Source: CAD feature listing. Evaluate the final solid. Frame: model axes, mm. A direction names the side the tool comes from. Round coordinates to 2 decimals unless told otherwise and drop trailing zeros. Write each loop counter-clockwise with the first axis right and the second up, starting at its lowest first coordinate (ties: lowest second). Pieces come first, ordered by that corner, then holes.
from build123d import *

# Parameters (mm, degrees)
F0_W     = 152.4
F0_H     = 127
F1_DEPTH = 50.8
F3_DEPTH = 101.6
F5_DEPTH = 25.4
F6_W     = 127
F6_H     = 50.8
F7_DEPTH = 127


with BuildPart() as f1:
    # F0 (on Front) → F1 (new body)
    with BuildSketch(Plane.XZ):
        with Locations((-6.594061, 23.633106)):
            Rectangle(F0_W, F0_H)
    extrude(amount=F1_DEPTH)

    # F2 (on face) → F3 (join)
    with BuildSketch(Plane.XZ.offset(50.8)):
        Polygon((18.805939, -14.466894), (69.605939, -14.466894), (69.605939, 87.133106), (-57.394061, 87.133106), (-57.394061, 61.733106), (18.805939, 61.733106), align=None)
    extrude(amount=F3_DEPTH)

    # F4 (on face) → F5 (join)
    with BuildSketch(Plane.XY.offset(87.133106)):
        Polygon((69.605939, 0), (-82.794061, 0), (-82.794061, -50.8), (-57.394061, -50.8), (-57.394061, -152.4), (69.605939, -152.4), align=None)
    extrude(amount=F5_DEPTH)

    # F6 (on face) → F7 (join)
    with BuildSketch(Plane.XY.offset(112.533106)):
        with Locations((6.105939, -127)):
            Rectangle(F6_W, F6_H)
    extrude(amount=F7_DEPTH)


solid = f1.part
1) Section query C-C on y = -57.5. Return the cut outline in (x, z), then the cut area to 3 significant figures.
Taken from the geometry:
outline: (-57.39, 61.73) - (18.81, 61.73) - (18.81, -14.47) - (69.61, -14.47) - (69.61, 112.53) - (-57.39, 112.53) - close
area: 10,300 mm2
2) Section query D-D on x = -61. Return the cut outline in (y, z).
Taken from the geometry:
outline: (-50.8, -39.87) - (0, -39.87) - (0, 112.53) - (-50.8, 112.53) - close
3) Material intervals for line 1 (Z direction, x = -25, y = -20.5); line 2 (Y direction, x = -71, z = -28); line 3 (X direction, y = -113.5, z = 3), sorted ascending.
Taken from the geometry:
line 1: z = -39.87 to 112.53
line 2: y = -50.8 to 0
line 3: x = 18.81 to 69.61
4) Reachability of faces 1 (the face through (-57.394, -114, 130)), 2 (the face through (5, -101.6, 175)), 3 (the face through (18.806, -101, 24)) from +Z, -Z, +X, -X, +Y, -Y: full face, straight path, thin tool, end or side. Return the list, or none.
Taken from the geometry:
face 1: +Z, -Z, -X, -Y
face 2: +Z, +X, -X, +Y
face 3: -Z, -X, -Y
5) Section query B-B on z = -9. Return the cut outline in (x, y).
Taken from the geometry:
outline: (-82.79, -50.8) - (18.81, -50.8) - (18.81, -152.4) - (69.61, -152.4) - (69.61, 0) - (-82.79, 0) - close
6) Section query A-A on x = -4. Return the cut outline in (y, z), then the cut area to 3 significant figures.
Taken from the geometry:
outline: (-152.4, 61.73) - (-50.8, 61.73) - (-50.8, -39.87) - (0, -39.87) - (0, 112.53) - (-101.6, 112.53) - (-101.6, 239.53) - (-152.4, 239.53) - close
area: 19,400 mm2
7) Contact query for flat-ended pins moving along their axis: P1, Ø1, axis at x = 42.5, y = -63.5, coming from the +Z side; P2, Ø2, axis at x = -41, y = -70, coming from the -Z side. Output: stop coordinate, or through.
Taken from the geometry:
P1: stops at z = 112.53
P2: stops at z = 61.73
